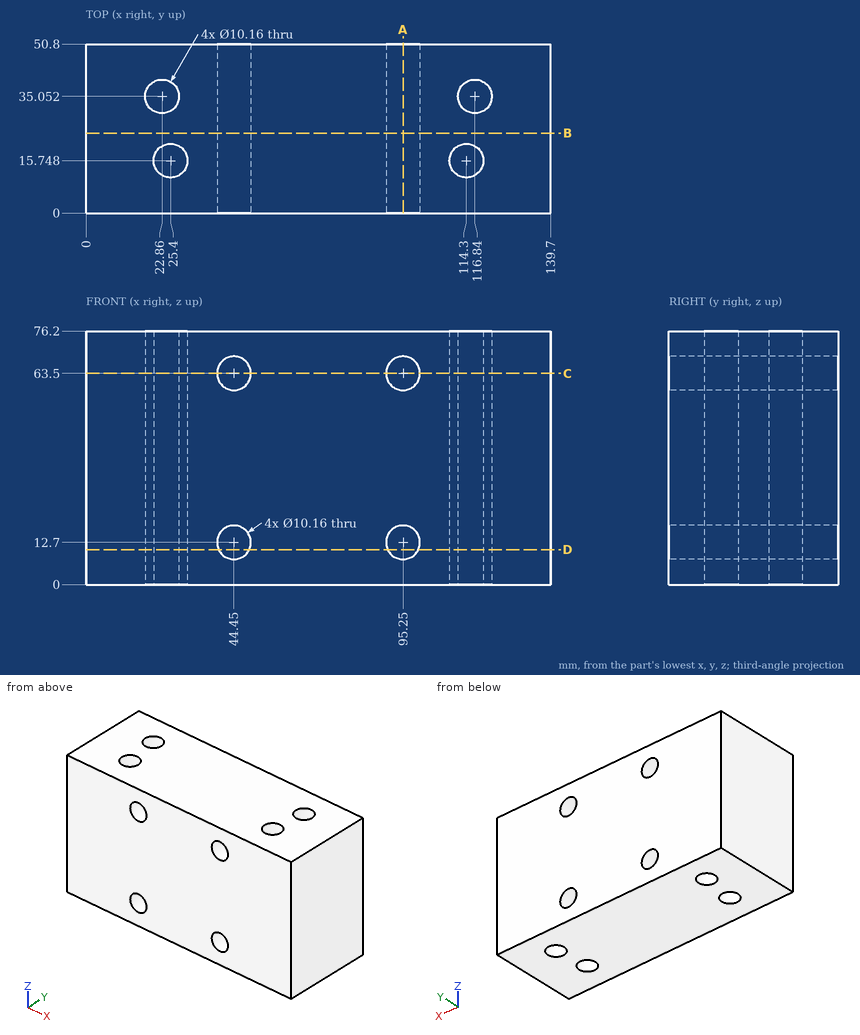
The drawing under review shows one solid part. Ordinate dimensions are in mm from its lowest x, y, z. Round coordinates to 2 decimals unless told otherwise and drop trailing zeros. Write each loop counter-clockwise with the first axis right and the second up, starting at its lowest first coordinate (ties: lowest second). Pieces come first, ordered by that corner, then holes. Notation, with made-up numbers: (0, 16.5) - (51, 16.5) arc R22 cw to (51, 48.5) - close; hole circle Ø2 at (58.25, -11.5). An arc over 180 degrees is marked (long way). Write each question's results on one line, items separated by ' | '.
Item 1: Take a section at B-B on y = 24. State the section outline as (x, z) points, then the cut area to 3 significant figures.
Calculated:
outline: (0, 0) - (139.7, 0) - (139.7, 76.2) - (0, 76.2) - close; hole circle Ø10.16 at (44.45, 12.7); hole circle Ø10.16 at (44.45, 63.5); hole circle Ø10.16 at (95.25, 12.7); hole circle Ø10.16 at (95.25, 63.5) | area: 10,300 mm^2
Item 2: To check wall thickness, follow line 1 along Z through (x, y) = (95.25, 18); line 2 along Z through (x, y) = (93, 4.5); line 3 along Y through (x, z) = (116, 23.5). State the ranges of each line that lie inside material, in increasing order. Write a range as from..to.
Calculated:
line 1: z = 0..7.62, 17.78..58.42, 68.58..76.2 | line 2: z = 0..8.15, 17.25..58.95, 68.05..76.2 | line 3: y = 0..10.96, 20.54..30.04, 40.06..50.8
Item 3: Take a section at D-D on z = 10.5. State the section outline as (x, y) points, then the cut area to 3 significant figures.
Calculated:
outline: (0, 0) - (39.87, 0) - (39.87, 50.8) - (0, 50.8) - close; (49.03, 0) - (90.67, 0) - (90.67, 50.8) - (49.03, 50.8) - close; (99.83, 0) - (139.7, 0) - (139.7, 50.8) - (99.83, 50.8) - close; hole circle Ø10.16 at (22.86, 35.05); hole circle Ø10.16 at (25.4, 15.75); hole circle Ø10.16 at (114.3, 15.75); hole circle Ø10.16 at (116.84, 35.05) | area: 5,840 mm^2
Item 4: Take a section at A-A on x = 95.25. State the section outline as (y, z) points.
Calculated:
outline: (0, 0) - (50.8, 0) - (50.8, 7.62) - (0, 7.62) - close; (0, 17.78) - (50.8, 17.78) - (50.8, 58.42) - (0, 58.42) - close; (0, 68.58) - (50.8, 68.58) - (50.8, 76.2) - (0, 76.2) - close
Item 5: Take a section at C-C on z = 63.5. State the section outline as (x, y) points, then the cut area to 3 significant figures.
Calculated:
outline: (0, 0) - (39.37, 0) - (39.37, 50.8) - (0, 50.8) - close; (49.53, 0) - (90.17, 0) - (90.17, 50.8) - (49.53, 50.8) - close; (100.33, 0) - (139.7, 0) - (139.7, 50.8) - (100.33, 50.8) - close; hole circle Ø10.16 at (22.86, 35.05); hole circle Ø10.16 at (25.4, 15.75); hole circle Ø10.16 at (114.3, 15.75); hole circle Ø10.16 at (116.84, 35.05) | area: 5,740 mm^2
